Model file for the job. Use its own axes, mm. Face numbers are marked on the shaded views. A direction names the side the tool comes from. Round coordinates to 2 decimals unless told otherwise and drop trailing zeros. Loops run counter-clockwise (first coordinate to the right, second up) from the corner with the lowest first, then second, coordinate; pieces in that order, holes last. Notation, with made-up numbers: M 49.5,-2 L 76.5,-2 A17 ccw 76.5,20 Z; hole C 11,80 d7. An arc over 180 degrees is marked long. Answer in a Markdown table with one row per item.
from build123d import *

# Parameters (mm, degrees)
SKETCH1_W           = 90
SKETCH1_H           = 70.15
SKETCH1_R           = 1.65
BOSS_EXTRUDE1_DEPTH = 15.45
SKETCH2_W           = 12.2
SKETCH2_H           = 12.46
BOSS_EXTRUDE2_DEPTH = 50


with BuildPart() as part:
    # Sketch1 → Boss-Extrude1 (new body)
    with BuildSketch(Plane(origin=(0, 0, 0), x_dir=(1, 0, 0), z_dir=(0, 1, 0))):
        Rectangle(SKETCH1_W, SKETCH1_H)
        with Locations(Location((-41.05, 31.125, 0), (0, 0, 270))):
            Circle(SKETCH1_R, mode=Mode.SUBTRACT)
        with Locations(Location((41.05, 31.125, 0), (0, 0, 270))):
            Circle(SKETCH1_R, mode=Mode.SUBTRACT)
        with Locations(Location((-41.05, -31.125, 0), (0, 0, 270))):
            Circle(SKETCH1_R, mode=Mode.SUBTRACT)
        with Locations(Location((41.05, -31.125, 0), (0, 0, 270))):
            Circle(SKETCH1_R, mode=Mode.SUBTRACT)
    extrude(amount=BOSS_EXTRUDE1_DEPTH)

    # Sketch2 → Boss-Extrude2 (add)
    with BuildSketch(Plane.XY.offset(35.075)):
        with Locations((-9.2, 6.23)):
            Rectangle(SKETCH2_W, SKETCH2_H)
    extrude(amount=BOSS_EXTRUDE2_DEPTH)


solid = part.part
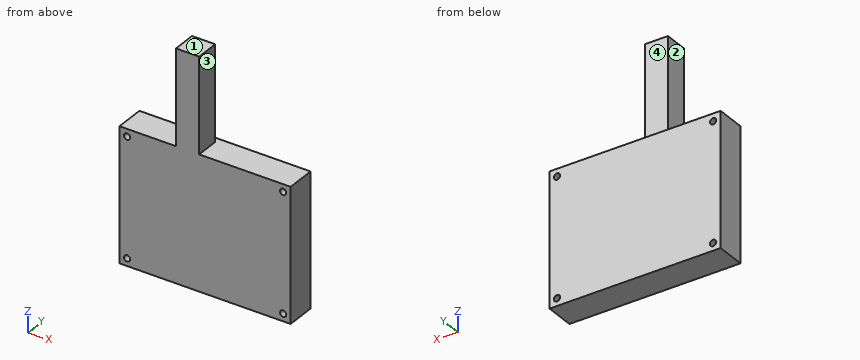
1. Wall check: probe 1 along X at (y, z) = (6, 30.5); probe 2 along Z at (x, y) = (17, 8.5) (3 decimals); probe 3 along X at (y, z) = (4.5, 53.5). Give the ranges that are in metal, low to high.
Verdict:
| item | result |
|---|---|
| probe 1 | x = -45 to -42.58, -39.52 to 39.52, 42.58 to 45 |
| probe 2 | z = -35.075 to 35.075 |
| probe 3 | x = -15.3 to -3.1 |
2. Saw through at C-C (z = 40). Write the cut outline in (x, y), and give its area (3 significant figures).
Verdict:
| item | result |
|---|---|
| outline | M -15.3,0 L -3.1,0 L -3.1,12.46 L -15.3,12.46 Z |
| area | 152 mm² |
3. Pin check, flat tips, straight feed: pin 1 (6 mm diameter, centred on y = 5.5, z = 67, fed in from -X); pin 2 (10 mm diameter, centred on x = -9, z = 61.5, fed in from +Y). Stop position of each tip, or through.
Verdict:
| item | result |
|---|---|
| pin 1 | stops at x = -15.3 |
| pin 2 | stops at y = 12.46 |
4. Saw through at B-B (y = 1.5). Write the cut outline in (x, z) (3 decimals), and give its area (3 significant figures).
Verdict:
| item | result |
|---|---|
| outline | M -45,-35.075 L 45,-35.075 L 45,35.075 L -3.1,35.075 L -3.1,85.075 L -15.3,85.075 L -15.3,35.075 L -45,35.075 Z; hole C -41.05,-31.125 d3.3; hole C -41.05,31.125 d3.3; hole C 41.05,-31.125 d3.3; hole C 41.05,31.125 d3.3 |
| area | 6,890 mm² |
5. Saw through at D-D (x = 4). Write the cut outline in (y, z) (3 decimals), and give its area (3 significant figures).
Verdict:
| item | result |
|---|---|
| outline | M 0,-35.075 L 15.45,-35.075 L 15.45,35.075 L 0,35.075 Z |
| area | 1,080 mm² |
6. Tool access for the marked faces 1, 2, 3 and 4: list every direction of +Z, -Z, +X, -X, +Y, -Y with a clear straight run to the whole face (end or side of a thin tool).
Verdict:
| item | result |
|---|---|
| face 1 | +Z, +X, -X, +Y, -Y |
| face 2 | +Z, -X, +Y, -Y |
| face 3 | +Z, +X, +Y, -Y |
| face 4 | +Z, +X, -X, +Y |
7. Saw through at A-A (x = 41.05). Write the cut outline in (y, z) (3 decimals), and give its area (3 significant figures).
Verdict:
| item | result |
|---|---|
| outline | M 0,-35.075 L 15.45,-35.075 L 15.45,-32.775 L 0,-32.775 Z; M 0,-29.475 L 15.45,-29.475 L 15.45,29.475 L 0,29.475 Z; M 0,32.775 L 15.45,32.775 L 15.45,35.075 L 0,35.075 Z |
| area | 982 mm² |
